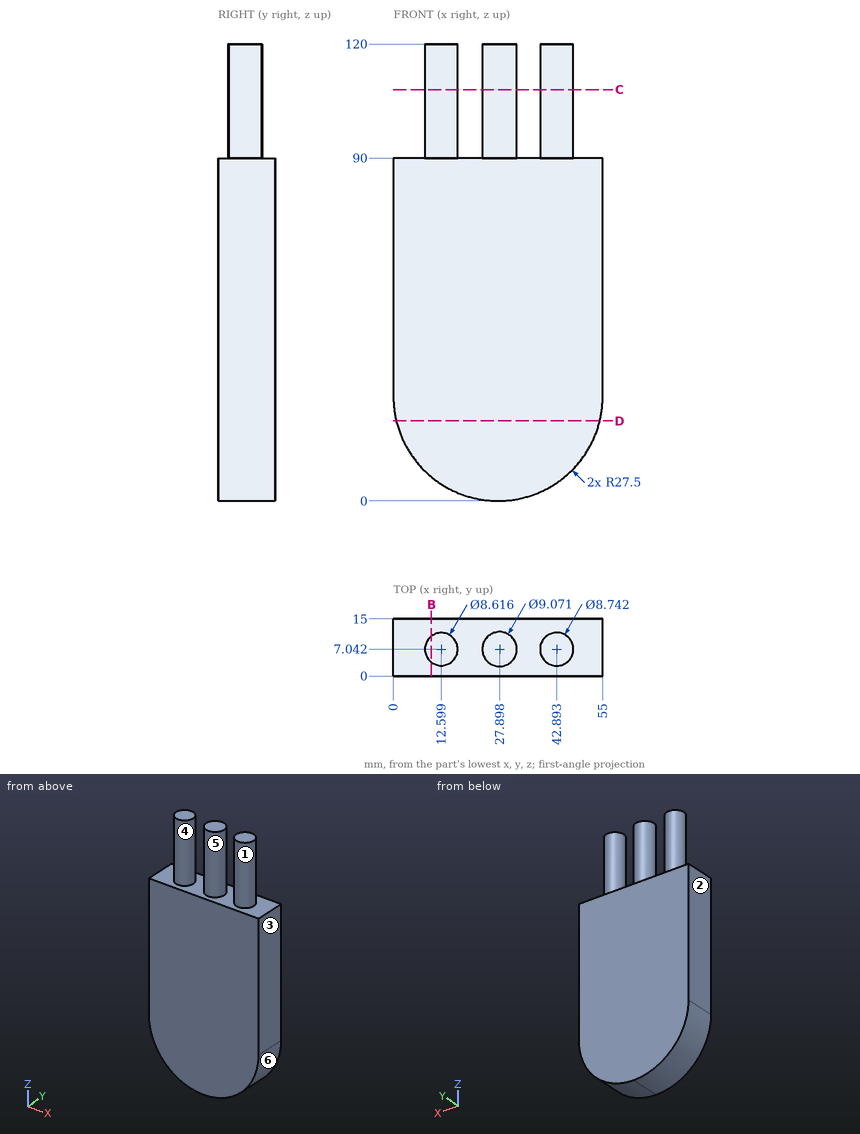
Drawing for the job (mm, zero at the part's lowest x, y, z). A direction names the side the tool comes from. Give positions to 0.01 mm unless a question says otherwise; leave off trailing zeros. Write each loop counter-clockwise with the first axis right and the second up, starting at its lowest first coordinate (ties: lowest second). Pieces come first, ordered by that corner, then holes. Notation, with made-up numbers: (16.5, -14) -> (50.5, -14) arc R19 cw to (50.5, -4) -> close; hole circle Ø3 at (0.5, 61.5). An arc over 180 degrees is marked (long way). Put each result on its own line as item: value. Start each with the question number.
Item 1: Cut at D-D (z = 21). List the corners of the cut face in (x, y).
Item 2: Cut at C-C (z = 108). List the corners of the cut face in (x, y) (1 decimal), then the cut area to 3 significant figures.
Item 3: Pull direction X, two halves, no side cores. Call the marked faces 1, 2, 3 and 4: pulls with the +X half, pulls with the -X half, needs draft (parallel to the pull), parting line crosses it, or undercut.
Item 4: Wall check: L1, parallel to X at y = 8, z = 90.5 (1 decimal); L2, parallel to Z at x = 26.5, y = 3.5; L3, parallel to X at y = 6.25, z = 110.5 (1 decimal). Give the ranges that are in metal, low to high. Write a range as [from, to].
Item 5: Pin check, flat tips, straight feed: pin 1 Ø5 at (x, y) = (39, 6) entering from -Z (1 decimal); pin 2 Ø6 at (x, y) = (6.5, 8.5) entering from -Z; pin 3 Ø3 at (x, y) = (40, 9.5) entering from -Z (1 decimal). Stop position of each tip, or through.
Item 6: Which spindle directions (+Z, -Z, +X, -X, +Y, -Y) get a long thin tool onto all of the face, cutting with end or side? Do the marked faces 5 and 6. Say none if no direction does.
Item 7: Cut at B-B (x = 10). List the corners of the cut face in (y, z) (1 decimal), then the cut area to 3 significant figures.
Answer list:
1. outline: (0.78, 0) -> (54.22, 0) -> (54.22, 15) -> (0.78, 15) -> close
2. outline: circle Ø8.6 at (12.6, 7); circle Ø9.1 at (27.9, 7); circle Ø8.7 at (42.9, 7)
2. area: 183 mm2
3. face 1: undercut
3. face 2: pulls with the -X half
3. face 3: pulls with the +X half
3. face 4: undercut
4. L1: x = [8.4, 16.8], [23.5, 32.3], [38.6, 47.2]
4. L2: z = [0.02, 120]
4. L3: x = [8.4, 16.8], [23.4, 32.4], [38.6, 47.2]
5. pin 1: stops at z = 1.5
5. pin 2: stops at z = 6.71
5. pin 3: stops at z = 2.3
6. face 5: +Z
6. face 6: -Z, +X, +Y, -Y
7. outline: (0, 6.3) -> (15, 6.3) -> (15, 90) -> (10.5, 90) -> (10.5, 120) -> (3.6, 120) -> (3.6, 90) -> (0, 90) -> close
7. area: 1,460 mm2
